Autodesk Inventor part; units mm, degrees
ref_plane "YZ Plane" through (0, 0, 0) normal (1, 0, 0) x (0, 1, 0)
ref_plane "XZ Plane" through (0, 0, 0) normal (0, 1, 0) x (-1, 0, 0)
ref_plane "XY Plane" through (0, 0, 0) normal (0, 0, 1) x (1, 0, 0)
sketch "Sketch1" plane through (0, 0, 0) normal (0, 1, 0) x (-1, 0, 0)
  line L0 (0, 0) -> (31.75, 0)
  line L1 (31.75, 0) -> (31.75, -3.175)
  line L2 (31.75, -3.175) -> (4.7625, -3.175)
  line L3 (4.7625, -3.175) -> (4.7625, -38.1)
  line L4 (4.7625, -38.1) -> (0, -38.1)
  line L5 (0, 0) -> (0, -38.1)
  point P0 (31.75, -1.5875)
  dimension "d1" = 3.175
  dimension "d2" = 31.75
  dimension "d3" = 38.1
  dimension "d4" = 4.7625
extrude "Extrusion1" add sketch "Sketch1" along normal blind 46.0375
sketch "Sketch2" plane through (-31.75, 0, 0) normal (0, 0, 1) x (1, 0, 0)
  line L0 (0, 0) -> (0, 46.0375)
  line L1 (31.75, 0) -> (31.75, 46.0375)
  line L2 (6.35, 5.334) -> (24.35, 5.334) construction
  line L3 (24.35, 5.334) -> (24.35, 38.334) construction
  line L4 (24.35, 38.334) -> (6.35, 38.334) construction
  line L5 (6.35, 38.334) -> (6.35, 5.334) construction
  circle A0 centre (24.35, 5.334) radius 1.625
  circle A1 centre (6.35, 38.334) radius 1.625
  circle A2 centre (24.35, 38.334) radius 1.625
  line L6 (0, 0) -> (31.75, 0)
  circle A3 centre (15.35, 14.334) radius 7.62
  dimension "d24" = 3.25
  dimension "d25" = 3.25
  dimension "d26" = 3.25
  dimension "d27" = 33
  dimension "d38" = 15.24
  dimension "d53" = 6.35
  dimension "d54" = 9
  dimension "d55" = 18
  dimension "d56" = 5.334
  dimension "d57" = 9
extrude "Extrusion2" cut sketch "Sketch2" against normal blind 46.0375
sketch "Sketch3" plane through (0, 46.0375, 0) normal (0, 1, 0) x (1, 0, 0)
  line L0 (0, 38.1) -> (-4.7625, 38.1)
  line L1 (-4.7625, 38.1) -> (-4.7625, 3.175)
  line L2 (-4.7625, 3.175) -> (-31.75, 3.175)
  line L3 (-31.75, 3.175) -> (-31.75, 0)
  line L4 (-31.75, 0) -> (0, 0)
  line L5 (0, 0) -> (0, 38.1)
  line L6 (-31.75, 3.175) -> (-4.7625, 38.1)
extrude "Extrusion3" add sketch "Sketch3" against normal blind 3.175 contours L1 L2 L6
sketch "Sketch4" plane through (-4.7625, 0, -38.1) normal (-1, 0, 0) x (0, 0, 1)
  circle A0 centre (28.575, 31.75) radius 2.159
  circle A1 centre (6.35, 6.35) radius 2.159
  line L0 (0, 0) -> (0, 42.8625)
  line L1 (0, 0) -> (34.925, 0)
  line L2 (34.925, 42.8625) -> (0, 42.8625)
  line L3 (34.925, 0) -> (34.925, 42.8625)
  circle A2 centre (28.575, 31.75) radius 4.3656
  point P0 (38.1, 0)
  dimension "d41" = 4.318
  dimension "d42" = 4.318
  dimension "d43" = 6.35
  dimension "d44" = 6.35
  dimension "d45" = 11.1125
  dimension "d47" = 6.35
  dimension "d50" = 8.7312
extrude "Extrusion4" cut sketch "Sketch4" against normal through all contours A0 | A1
fillet "Fillet1" radius 3.175 1 edges at (-4.7625, 42.8625, -20.6375)
properties part number "Motor Mount V1_3DPrint"
Input: part model. Units: mm. Frame: model coordinates. A direction names the side the tool comes from. Give positions to 0.01 mm unless a question says otherwise; leave off trailing zeros. Write each loop counter-clockwise with the first axis right and the second up, starting at its lowest first coordinate (ties: lowest second). Pieces come first, ordered by that corner, then holes. Notation, with made-up numbers: (89, 13.5) - (148, 13.5) arc R23 ccw to (148, 21.5) - close; hole circle Ø2 at (-22, 15). An arc over 180 degrees is marked (long way). Write item = value, one per line. Start each with the question number.
1) Cut plane D-D (y = 37.5). Give the number of separate pieces and of enclosed holes in the cut face, and give its area (3 significant figures).
2) Pin query (flat end, axial travel): pin 1 (19 mm diameter, centred on x = -21.5, z = -20.5, fed in from -Y); pin 2 (8 mm diameter, centred on y = 18.5, z = -34, fed in from -X); pin 3 (12 mm diameter, centred on x = -22.5, y = 20.5, fed in from -Z) (3 decimals). Return the tip coordinate at first contact, or that it passes through.
3) Reachability of faces 4 (the face through (-5.67, 41.91, -20.39)), 5 (the face through (-22.45, 9.7, -1.57)) from +Z, -Z, +X, -X, +Y, -Y: full face, straight path, thin tool, end or side. Return the list, or none.
4) Cut plane B-B (x = -25.4). Return loops of the section in (y, z) (1 decimal).
5) Material intervals for L1, parallel to Y at x = -7.4, z = -1.6; L2, parallel to Y at x = -16.4, z = -1.7; L3, parallel to Z at x = -7, y = 28.5 (3 decimals), sorted ascending. Write a range as [from, to].
6) Draft query along Y for faces 1 (the face through (-7.752, 36.748, -1.565)), 2 (the face through (-2, 23, -38.1)), 3 (the face through (-13, 46.038, -15)). Return one class per face: pulls with the +Y half, pulls with the -Y half, needs draft (parallel to the pull), parting line crosses it, or undercut.
Answers follow:
q1.separate_pieces = 3
q1.enclosed_holes = 0
q1.area = 249 mm^2
q2.pin_1 = 42.86
q2.pin_2 = -4.76
q2.pin_3 = -3.175
q3.face_4 = -Z, -X, -Y
q3.face_5 = +Z, -Z
q4.outline = (0, -3.2) - (36.7, -3.2) - (36.7, 0) - (0, 0) - close; (40, -3.2) - (42.9, -3.2) - (42.9, -11.4) - (46, -11.4) - (46, 0) - (40, 0) - close
q5.L1 = [0, 3.71], [6.96, 36.71], [39.96, 46.04]
q5.L2 = [0, 6.71], [21.95, 46.04]
q5.L3 = [-3.175, 0]
q6.face_1 = undercut
q6.face_2 = needs draft
q6.face_3 = pulls with the +Y half
